Build history of the part. All positions in model axes, mm. A direction names the side the tool comes from. Round coordinates to 2 decimals unless told otherwise and drop trailing zeros. Loops run counter-clockwise (first coordinate to the right, second up) from the corner with the lowest first, then second, coordinate; pieces in that order, holes last. Notation, with made-up numbers: M 57,55.25 L 95,55.25 A27 cw 95,71.25 Z; hole C 27.25,43.25 d7. An arc over 180 degrees is marked long. One line per item, written item: value.
```python
from build123d import *

# Parameters (mm, degrees)
SKETCH_1_W      = 41
SKETCH_1_H      = 20
EXTRUDE_1_DEPTH = 42
SKETCH_3_W      = 2.5
SKETCH_3_H      = 20
EXTRUDE_2_DEPTH = 7
SKETCH_4_W      = 2.5
SKETCH_4_H      = 20
EXTRUDE_3_DEPTH = 7
SKETCH_5_R      = 2.95
EXTRUDE_4_DEPTH = 6


with BuildPart() as part:
    # ｽｹｯﾁ1 → ﾎﾞｽ - 押し出し1 (new body)
    with BuildSketch(Plane.XY):
        with Locations((-24.251560295, -13.435714286)):
            Rectangle(SKETCH_1_W, SKETCH_1_H)
    extrude(amount=EXTRUDE_1_DEPTH)

    # ｽｹｯﾁ3 → ﾎﾞｽ - 押し出し2 (add)
    with BuildSketch(Plane(origin=(-3.751560295, 0, 0), x_dir=(0, 0, -1), z_dir=(1, 0, 0))):
        with Locations((-35.25, -13.435714286)):
            Rectangle(SKETCH_3_W, SKETCH_3_H)
    extrude(amount=EXTRUDE_2_DEPTH)

    # ｽｹｯﾁ4 → ﾎﾞｽ - 押し出し3 (add)
    with BuildSketch(Plane.ZY.offset(44.751560295)):
        with Locations((35.25, -13.435714286)):
            Rectangle(SKETCH_4_W, SKETCH_4_H)
    extrude(amount=EXTRUDE_3_DEPTH)

    # ｽｹｯﾁ5 → ﾎﾞｽ - 押し出し4 (add)
    with BuildSketch(Plane.XY.offset(42)):
        with Locations((-34.751560295, -13.435714286)):
            Circle(SKETCH_5_R)
    extrude(amount=EXTRUDE_4_DEPTH)


solid = part.part
```
Item 1: Wall check: line 1 along Z through (x, y) = (-8.5, -9.5); line 2 along X through (y, z) = (-6.25, 3); line 3 along Z through (x, y) = (-3, -5.75). Give the ranges that are in metal, low to high.
Check values:
line 1: z = 0 to 42
line 2: x = -44.75 to -3.75
line 3: z = 34 to 36.5
Item 2: Slice it at D-D, the plane x = -48. Give the cut face in (y, z).
Check values:
outline: M -23.44,34 L -3.44,34 L -3.44,36.5 L -23.44,36.5 Z
Item 3: Drop flat-ended pins along their axis: P1, Ø1, axis at x = -39.5, y = -17.5, coming from the +Z side; P2, Ø5.5, axis at x = 1, y = -11, coming from the -Z side; P3, Ø3, axis at y = -16, z = 39, coming from the +X side. Give the stop position or say it passes through.
Check values:
P1: stops at z = 42
P2: stops at z = 34
P3: stops at x = -3.75
Item 4: Slice it at C-C, the plane z = 31. Give the cut face in (x, y).
Check values:
outline: M -44.75,-23.44 L -3.75,-23.44 L -3.75,-3.44 L -44.75,-3.44 Z
Item 5: Slice it at A-A, the plane y = -21.75. Give the cut face in (x, z), and give its area (3 significant figures).
Check values:
outline: M -51.75,34 L -44.75,34 L -44.75,0 L -3.75,0 L -3.75,34 L 3.25,34 L 3.25,36.5 L -3.75,36.5 L -3.75,42 L -44.75,42 L -44.75,36.5 L -51.75,36.5 Z
area: 1,760 mm2
Item 6: Slice it at B-B, the plane x = -32.5. Give the cut face in (y, z).
Check values:
outline: M -23.44,0 L -3.44,0 L -3.44,42 L -11.53,42 L -11.53,48 L -15.34,48 L -15.34,42 L -23.44,42 Z
Item 7: Which spindle directions (+Z, -Z, +X, -X, +Y, -Y) get a long thin tool onto all of the face, cutting with end or side? Do faces 1 (the face through (0, -14, 36.5)), 2 (the face through (-48, -14, 36.5)), 3 (the face through (-48, -14, 34)). Say none if no direction does.
Check values:
face 1: +Z, +X, +Y, -Y
face 2: +Z, -X, +Y, -Y
face 3: -Z, -X, +Y, -Y
